For this review, take the finished solid that the model builds, in its own axes (mm). A direction names the side the tool comes from. Coordinates: 2 decimals unless noted, no trailing zeros. Write each loop counter-clockwise with the first axis right and the second up, starting at its lowest first coordinate (ties: lowest second). Pieces come first, ordered by that corner, then holes.
```python
from build123d import *

# Parameters (mm, degrees)
F0_R     = 6
F1_DEPTH = 67
F3_R     = 10.75
F4_DEPTH = 22
F5_W     = 26.495327
F5_H     = 31.794394
F5_W_2   = 19
F5_H_2   = 24.700004
F6_DEPTH = 6
F7_SIZE  = 1


with BuildPart() as f1:
    # F0 (on Front) → F1 (new body)
    with BuildSketch(Plane.XZ):
        Circle(F0_R)
    extrude(amount=F1_DEPTH)

    # F3 (on offset) → F4 (join)
    with BuildSketch(Plane.XZ.offset(52)):
        Circle(F3_R)
    extrude(amount=-F4_DEPTH)

    # F5 (on face) → F6 (cut)
    with BuildSketch(Plane(origin=(0, -30, 0), x_dir=(-1, 0, 0), z_dir=(0, 1, 0))):
        with Locations((-0.883178, -0.441589)):
            Rectangle(F5_W, F5_H)
        with Locations((2e-06, -0.147196)):
            Rectangle(F5_W_2, F5_H_2, mode=Mode.SUBTRACT)
    extrude(amount=-F6_DEPTH, mode=Mode.SUBTRACT)

    # F7
    f7_edges = [f1.edges().sort_by_distance(p)[0] for p in [
        (-6, -67, 0),
        (-6, 0, 0),
        (-4e-06, -30, -10.75),
        (-4e-06, -30, 10.75),
    ]]
    chamfer(f7_edges, length=F7_SIZE)


solid = f1.part
```
Q1. Clearance check with flat-ended pins moving along their axes: pin 1 Ø4 at (x, z) = (6.5, 3) entering from -Y; pin 2 Ø1.5 at (y, z) = (-47, 2) entering from -X; pin 3 Ø1 at (x, z) = (10.5, 1.5) entering from +Y; pin 4 Ø9.5 at (x, z) = (3.5, -4) entering from +Y. State where each tip first meets the part, or that it passes through.
Ans:
pin 1: stops at y = -66.84
pin 2: stops at x = -10.68
pin 3: stops at y = -36
pin 4: stops at y = 0
Q2. Add section C-C (y = -55). State the section outline as (x, z) points, then the cut area to 3 significant figures.
Ans:
outline: circle Ø12 at (0, 0)
area: 113 mm2
Q3. Add section B-B (x = 0). State the section outline as (y, z) points.
Ans:
outline: (-67, -5) - (-66, -6) - (-52, -6) - (-52, -10.75) - (-31, -10.75) - (-30, -9.75) - (-30, -6) - (-1, -6) - (0, -5) - (0, 5) - (-1, 6) - (-30, 6) - (-30, 9.75) - (-31, 10.75) - (-52, 10.75) - (-52, 6) - (-66, 6) - (-67, 5) - close
Q4. Tool access review of faces 1 (the flat face through (9.5, -33, 0)), 2 (the flat face through (-10, -36, 0)), 3 (the flat face through (-4.4, -30, 4.5)), 4 (the cylindrical face through (-6, -59, 0)), 5 (the flat face through (0, -67, 0)): name each direction out of +Z, -Z, +X, -X, +Y, -Y from which nothing blocks a thin tool from reaching the whole face with its end or side.
Ans:
face 1: +Z, -Z, +X, +Y
face 2: +Z, -Z, -X, +Y
face 3: +Y
face 4: -Y
face 5: +Z, -Z, +X, -X, -Y
Q5. For probe 1 along Y at (x, z) = (-6, -2.75); probe 2 along X at (y, z) = (-35, -3); probe 3 along Z at (x, y) = (5, -42), list the stretches that pass through material, from the lowest coordinate up.
Ans:
probe 1: y = -52 to -30
probe 2: x = -9.5 to 9.5
probe 3: z = -9.52 to 9.52
Q6. Add section A-A (z = 0). State the section outline as (x, y) points, then the cut area to 3 significant figures.
Ans:
outline: (-10.75, -52) - (-6, -52) - (-6, -66) - (-5, -67) - (5, -67) - (6, -66) - (6, -52) - (10.75, -52) - (10.75, -36) - (9.5, -36) - (9.5, -30) - (6, -30) - (6, -1) - (5, 0) - (-5, 0) - (-6, -1) - (-6, -30) - (-9.5, -30) - (-9.5, -36) - (-10.75, -36) - close
area: 996 mm2
